Geometry: final body of the model. Coordinates: model frame, mm. A direction names the side the tool comes from. Give positions to 0.01 mm unless a question says otherwise; leave off trailing zeros. Answer in a Markdown table with one row per item. Add a question column.
from build123d import *
from build123d.topology import SkipClean

# Parameters (mm, degrees)
REVOLVE1_ANGLE       = 60
CUT_EXTRUDE1_DEPTH   = 151.38335158
BOSS_EXTRUDE1_DEPTH  = 12
BOSS_EXTRUDE2_DEPTH  = 7.5
CUT_EXTRUDE2_DEPTH   = 4.5
CHAMFER2_SIZE        = 4.5
CHAMFER5_SIZE2       = 3
CHAMFER5_SIZE        = 4.5
CHAMFER3_SIZE        = 1.5
CUT_REVOLVE1_ANGLE   = 90
CHAMFER4_SIZE        = 4.5
MIRROR4_COPY_1_ANGLE = 90
CHAMFER1_SIZE        = 1


with BuildPart() as part:
    # Sketch2 → Revolve1 (revolve)
    with BuildSketch(Plane.XY):
        Polygon((-16, 12), (-20, 12), (-20, 0), (20, 0), (20, 12), (16, 12), (16, 9), (10, 9), (10, 12), (-10, 12), (-10, 9), (-16, 9), align=None)
    revolve(axis=Axis((129.9038106, 0, 0), (0, -1, 0)), revolution_arc=REVOLVE1_ANGLE)

    # Sketch3 → Cut-Extrude1 (cut, through all)
    with BuildSketch(Plane(origin=(0, 12, 0), x_dir=(1, 0, 0), z_dir=(0, 1, 0))):
        with BuildLine():
            ThreePointArc((6.5, 11.5), (-3.122498999, 17.200877125), (-3.5, 6.022774425))
            Line((-3.5, 6.022774425), (-3.5, 11.5))
            Line((-3.5, 11.5), (3.5, 11.5))
            Line((3.5, 11.5), (3.5, 6.022774425))
            ThreePointArc((3.5, 6.022774425), (5.700877125, 8.377501001), (6.5, 11.5))
        make_face()
        with BuildLine():
            Line((-3.5, 11.5), (-3.5, 6.022774425))
            ThreePointArc((-3.5, 6.022774425), (0, 5), (3.5, 6.022774425))
            Line((3.5, 6.022774425), (3.5, 11.5))
            Line((3.5, 11.5), (-3.5, 11.5))
        make_face()
        with BuildLine():
            Line((-3.5, 6.022774425), (-3.5, 0))
            Line((-3.5, 0), (3.5, 0))
            Line((3.5, 0), (3.5, 6.022774425))
            ThreePointArc((3.5, 6.022774425), (0, 5), (-3.5, 6.022774425))
        make_face()
    extrude(amount=-CUT_EXTRUDE1_DEPTH, mode=Mode.SUBTRACT)



with BuildPart() as body_2:
    # Sketch4 → Boss-Extrude1 (new body)
    with BuildSketch(Plane(origin=(0, 12, 0), x_dir=(1, 0, 0), z_dir=(0, 1, 0))):
        with BuildLine():
            ThreePointArc((68.937586537, 117.687885509), (69.715045021, 115.250000028), (71.437586537, 113.35775849))
            Line((71.437586537, 113.35775849), (76.161197444, 116.084936519))
            Line((76.161197444, 116.084936519), (73.661197444, 120.415063537))
            Line((73.661197444, 120.415063537), (68.937586537, 117.687885509))
        make_face()
        with BuildLine():
            Line((76.161197444, 116.084936519), (71.437586537, 113.35775849))
            ThreePointArc((71.437586537, 113.35775849), (77.66422619, 112.918880753), (80.911197444, 118.250000028))
            ThreePointArc((80.911197444, 118.250000028), (74.629830638, 124.243399124), (68.937586537, 117.687885509))
            Line((68.937586537, 117.687885509), (73.661197444, 120.415063537))
            Line((73.661197444, 120.415063537), (76.161197444, 116.084936519))
        make_face()
    extrude(amount=-BOSS_EXTRUDE1_DEPTH)


with BuildPart() as part_1:
    add(part.part)

    add(body_2.part)  # Boss-Extrude2 merges body 2
    # Sketch4<3> → Boss-Extrude2 (add)
    with BuildSketch(Plane(origin=(0, 12, 0), x_dir=(1, 0, 0), z_dir=(0, 1, 0))):
        with BuildLine():
            Line((63.7019053, 114.665063537), (66.2019053, 110.334936519))
            Line((66.2019053, 110.334936519), (71.437586537, 113.35775849))
            ThreePointArc((71.437586537, 113.35775849), (69.715045021, 115.250000028), (68.937586537, 117.687885509))
            Line((68.937586537, 117.687885509), (63.7019053, 114.665063537))
        make_face()
    extrude(amount=-BOSS_EXTRUDE2_DEPTH)

    # Sketch4<5> → Cut-Extrude2 (cut)
    with SkipClean():  # the faces are left unmerged after this step: merging them gives an invalid solid
        with BuildSketch(Plane(origin=(0, 12, 0), x_dir=(1, 0, 0), z_dir=(0, 1, 0))):
            with BuildLine():
                Line((63.7019053, 114.665063537), (66.2019053, 110.334936519))
                Line((66.2019053, 110.334936519), (71.437586537, 113.35775849))
                ThreePointArc((71.437586537, 113.35775849), (69.715045021, 115.250000028), (68.937586537, 117.687885509))
                Line((68.937586537, 117.687885509), (63.7019053, 114.665063537))
            make_face()
        extrude(amount=-CUT_EXTRUDE2_DEPTH, mode=Mode.SUBTRACT)

    # Chamfer2
    chamfer2_edges = [part_1.edges().sort_by_distance(p)[0] for p in [
        (80.107349866, 12, -121.250000028),
    ]]
    chamfer(chamfer2_edges, length=CHAMFER2_SIZE - 0.0001)  # a hair under: the kernel refuses the full size

    # Chamfer5
    chamfer5_edges = [part_1.edges().sort_by_distance(p)[0] for p in [
        (80.88480835, 0, -118.812114547),
    ]]
    chamfer5_side = [part_1.faces().sort_by_distance(p)[0] for p in [
        (80.88480835, 0.06, -118.812114547),
    ]]
    chamfer(chamfer5_edges, length=CHAMFER5_SIZE - 0.0001, length2=CHAMFER5_SIZE2 - 0.0001, reference=chamfer5_side[0])  # a hair under: the kernel refuses the full size

    # Chamfer3
    chamfer3_edges = [part_1.edges().sort_by_distance(p)[0] for p in [
        (0, 0, -18),
        (3.5, 0, -3.011387212),
        (-3.5, 12, -3.011387212),
        (-3.5, 0, -3.011387212),
        (0, 12, -18),
        (3.5, 12, -3.011387212),
    ]]
    chamfer(chamfer3_edges, length=CHAMFER3_SIZE)

    # Sketch17 → Cut-Revolve1 (revolve, cut)
    with BuildSketch(Plane(origin=(-33.72595265, 0, -58.415063523), x_dir=(-0.8660254037844378, 0, 0.5000000000000017), z_dir=(-0.5000000000000016, -1.1564823173178769e-15, -0.8660254037844377))):
        Polygon((-118.545643971, 10.545643943), (-118.545643971, 0), (-108.000000028, 0), align=None)
    cut_revolve1 = revolve(axis=Axis((38.154155888, -1.265151723, -99.915063537), (0, 1, 0)), revolution_arc=CUT_REVOLVE1_ANGLE, mode=Mode.SUBTRACT)

    # Mirror1: Cut-Revolve1 across plane
    add(cut_revolve1.mirror(Plane(origin=(-32.47595265, 0, -56.250000014), x_dir=(-0.866025403784439, -2.003086131649547e-15, 0.49999999999999933), z_dir=(-0.4999999999999994, -1.1564823173178701e-15, -0.866025403784439))), mode=Mode.SUBTRACT)

    # Chamfer4
    chamfer4_edges = [part_1.edges().sort_by_distance(p)[0] for p in [
        (64.9519053, 0, -112.500000028),
    ]]
    chamfer(chamfer4_edges, length=CHAMFER4_SIZE - 0.0001)  # a hair under: the kernel refuses the full size

    # Mirror4: Cut-Revolve1 across plane
    add(cut_revolve1.mirror(Plane(origin=(32.47595265, 0, -56.250000014), x_dir=(0.8660254037844382, 0, 0.5000000000000009), z_dir=(0.5000000000000009, 0, -0.8660254037844382))), mode=Mode.SUBTRACT)

    # Mirror4 copy 1 sketch → Mirror4 copy 1 (revolve, cut)
    with BuildSketch(Plane(origin=(2.5, 0, -112.500000028), x_dir=(0, 0, -1), z_dir=(1, 0, 0))):
        Polygon((-118.545643971, 10.545643943), (-118.545643971, 0), (-108.000000028, 0), align=None)
    revolve(axis=Axis((2.5, -1.265151723, -29.5), (0, 1, 0)), revolution_arc=MIRROR4_COPY_1_ANGLE, mode=Mode.SUBTRACT)

    # Chamfer1
    chamfer1_edges = [part_1.edges().sort_by_distance(p)[0] for p in [
        (0.083302496, 0, -74.9519053),
        (34.724318648, 0, -54.9519053),
        (-3.5, 7.508472143, 0),
        (3.5, 7.508472143, 0),
        (3.547404111, 12, -72.9519053),
        (8.743556534, 12, -69.9519053),
        (26.06406461, 12, -59.9519053),
        (31.260217033, 12, -56.9519053),
        (34.724318648, 12, -54.9519053),
        (0.083302496, 12, -74.9519053),
    ]]
    chamfer(chamfer1_edges, length=CHAMFER1_SIZE)


solid = part_1.part
(1) Draft query along Z for faces 5 (the flat face through (-11, 8, 0)), 6 (the flat face through (66.36, 6.02, -116.2)), 7 (the cylindrical face through (30.845, 9.986, -56.227)), 8 (the flat face through (30, 9, -56)). Return one class per face: +Z half, -Z half, draft (parallel to the pull), parting line (faces both ways), or undercut.
(2) Material intervals for line 1 along X through (y, z) = (10, -56.5); line 2 along Z through (x, y) = (52, 10.5); line 3 along Z through (x, y) = (75.5, 7.5), sorted ascending. Write a range as from..to.
(3) Reachability of faces 1 (the cylindrical face through (8.234, 9.986, -69.062)), 2 (the flat face through (-3.5, 6, -4)), 3 (the flat face through (68.783, 6.021, -111.825)), 4 (the cylindrical face through (-0.46, 5.93, -74)) from +Z, -Z, +X, -X, +Y, -Y: full face, straight path, thin tool, end or side. Return the list, or none.
(4) Pin query (flat end, axial travel): pin 1 Ø3 at (x, z) = (29, -101) entering from +Y; pin 2 Ø1.5 at (y, z) = (8, -3) entering from -X; pin 3 Ø3 at (x, y) = (37.5, 7.5) entering from +Z. Return the tip coordinate at first contact, or that it passes through.
Answer list:
| question | item | result |
|---|---|---|
| 1 | face 5 | +Z half |
| 1 | face 6 | -Z half |
| 1 | face 7 | undercut |
| 1 | face 8 | undercut |
| 2 | line 1 | x = -8.94..-4.62, 1.92..24.15, 31..35.64 |
| 2 | line 2 | z = -128.07..-123.36, -116.21..-91.15, -83.1..-77.52 |
| 2 | line 3 | z = -124.22..-112.28 |
| 3 | face 1 | +Y |
| 3 | face 2 | +Z, +Y, -Y |
| 3 | face 3 | +Y, -Y |
| 3 | face 4 | -Z, -X, +Y, -Y |
| 4 | pin 1 | stops at y = 9 |
| 4 | pin 2 | stops at x = -19.98 |
| 4 | pin 3 | stops at z = -57.1 |
